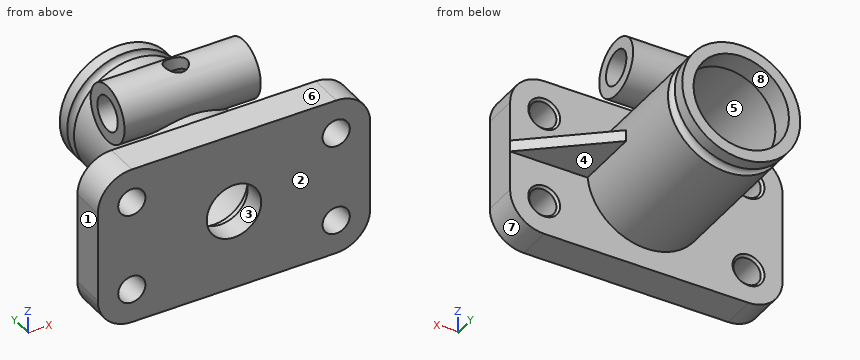
from build123d import *

# Parameters (mm, degrees)
SKETCH1_W                    = 120
SKETCH1_H                    = 70
BOSS_EXTRUDE1_DEPTH          = 15
SKETCH2_R                    = 26
BOSS_EXTRUDE2_DEPTH          = 70
SKETCH8_R                    = 2.5
BOSS_EXTRUDE3_DEPTH          = 2.5
SKETCH10_R                   = 12.5
BOSS_EXTRUDE4_DEPTH          = 60
SKETCH11_R                   = 23
CUT_EXTRUDE1_DEPTH           = 60
HOLE2_D                      = 15
SKETCH14_R                   = 5
CUT_EXTRUDE2_DEPTH           = 60
FILLET1_R                    = 15
M14_TAPPED_HOLE1_D           = 12
M14_TAPPED_HOLE1_CSINK_D     = 14.05
M14_TAPPED_HOLE1_CSINK_ANGLE = 90


with BuildPart() as part:
    # Sketch1 → Boss-Extrude1 (new body)
    with BuildSketch(Plane(origin=(0, 0, 0), x_dir=(1, 0, 0), z_dir=(0, 1, 0))):
        Rectangle(SKETCH1_W, SKETCH1_H)
    extrude(amount=BOSS_EXTRUDE1_DEPTH)

    # Sketch2 → Boss-Extrude2 (add)
    with BuildSketch(Plane(origin=(0, 15, 0), x_dir=(1, 0, 0), z_dir=(0, 1, 0))):
        with Locations(Location((0, 0, 0), (0, 0, 270))):
            Circle(SKETCH2_R)
    extrude(amount=BOSS_EXTRUDE2_DEPTH)

    # Sketch7 → Cut-Revolve2 (revolve, cut)
    with BuildSketch(Plane.XY, mode=Mode.PRIVATE) as cut_revolve2_sk:
        Polygon((0, 0), (0, 85), (21, 85), (21, 65), (23, 65), (23, 15), (15, 15), (15, 10), (12, 10), (12, 0), align=None)
    revolve(cut_revolve2_sk.sketch.rotate(Axis((0, 0, 0), (0, 1, 0)), 90), axis=Axis((0, 0, 0), (0, 1, 0)), mode=Mode.SUBTRACT)

    # Sketch8 → Cut-Revolve3 (revolve, cut)
    with BuildSketch(Plane.XY, mode=Mode.PRIVATE) as cut_revolve3_sk:
        with Locations((26, 77)):
            Circle(SKETCH8_R)
    revolve(cut_revolve3_sk.sketch.rotate(Axis((0, 0, 0), (0, 1, 0)), 90), axis=Axis((0, 0, 0), (0, 1, 0)), mode=Mode.SUBTRACT)

    # Sketch9 → Boss-Extrude3 (add, symmetric)
    with BuildSketch(Plane.XY):
        Polygon((24, 45), (60, 15), (24, 15), align=None)
    extrude(amount=BOSS_EXTRUDE3_DEPTH, both=True)

    # Sketch10 → Boss-Extrude4 (add)
    with BuildSketch(Plane(origin=(30, 0, 0), x_dir=(0, 0, -1), z_dir=(1, 0, 0))):
        with Locations((-30, 43)):
            Circle(SKETCH10_R)
    extrude(amount=-BOSS_EXTRUDE4_DEPTH)

    # Sketch11 → Cut-Extrude1 (cut)
    with BuildSketch(Plane(origin=(0, 15, 0), x_dir=(1, 0, 0), z_dir=(0, 1, 0))):
        with Locations(Location((0, 0, 0), (0, 0, 90))):
            Circle(SKETCH11_R)
    extrude(amount=CUT_EXTRUDE1_DEPTH, mode=Mode.SUBTRACT)

    # Hole2 (through all)
    with Locations(Plane(origin=(30, 0, 0), x_dir=(0, 0, -1), z_dir=(1, 0, 0))):
        with Locations((-30, 43)):
            Hole(HOLE2_D / 2)

    # Sketch14 → Cut-Extrude2 (cut)
    with BuildSketch(Plane.XY):
        with Locations(Location((0, 43, 0), (0, 0, 180))):
            Circle(SKETCH14_R)
    extrude(amount=CUT_EXTRUDE2_DEPTH, mode=Mode.SUBTRACT)

    # Fillet1
    fillet1_edges = [part.edges().sort_by_distance(p)[0] for p in [
        (-60, 7.5, -35),
        (60, 7.5, -35),
        (60, 7.5, 35),
        (-60, 7.5, 35),
    ]]
    fillet(fillet1_edges, radius=FILLET1_R)

    # M14 Tapped Hole1 (through all)
    with Locations(Plane(origin=(0, 15, 0), x_dir=(1, 0, 0), z_dir=(0, 1, 0))):
        with Locations((45, -20), (45, 20), (-45, 20), (-45, -20)):
            CounterSinkHole(M14_TAPPED_HOLE1_D / 2, M14_TAPPED_HOLE1_CSINK_D / 2, counter_sink_angle=M14_TAPPED_HOLE1_CSINK_ANGLE)


solid = part.part
Here's how the part is built. I have some questions about the finished solid (model axes, mm). Face numbers are marked on the shaded views. A direction names the side the tool comes from. Give positions to 0.01 mm unless a question says otherwise; leave off trailing zeros. Loops run counter-clockwise (first coordinate to the right, second up) from the corner with the lowest first, then second, coordinate; pieces in that order, holes last. Notation, with made-up numbers: (10, 51) -> (38, 51) arc R16 cw to (38, 72) -> close; hole circle Ø7 at (-17, -20). An arc over 180 degrees is marked (long way). One line per item, written item: value.
Q1. Suppose I cut it at B-B on z = 0. Please give me the cut outline in (x, y), then the cut area to 3 significant figures.
Answers follow:
outline: (-60, 0) -> (-12, 0) -> (-12, 10) -> (-15, 10) -> (-15, 15) -> (-23, 15) -> (-23, 75) -> (-21, 75) -> (-21, 85) -> (-26, 85) -> (-26, 79.5) arc R2.5 cw to (-26, 74.5) -> (-26, 15) -> (-60, 15) -> close; (12, 0) -> (60, 0) -> (60, 15) -> (26, 43.33) -> (26, 74.5) arc R2.5 cw to (26, 79.5) -> (26, 85) -> (21, 85) -> (21, 75) -> (23, 75) -> (23, 15) -> (15, 15) -> (15, 10) -> (12, 10) -> close
area: 2,330 mm^2
Q2. Suppose I cut it at A-A on y = 6.5. Please give me the cut outline in (x, z), then the cut area to 3 significant figures.
Answers follow:
outline: (-60, -20) arc R15 ccw to (-45, -35) -> (45, -35) arc R15 ccw to (60, -20) -> (60, 20) arc R15 ccw to (45, 35) -> (-45, 35) arc R15 ccw to (-60, 20) -> close; hole circle Ø12 at (-45, -20); hole circle Ø12 at (-45, 20); hole circle Ø24 at (0, 0); hole circle Ø12 at (45, -20); hole circle Ø12 at (45, 20)
area: 7,300 mm^2
Q3. On a 3-axis mill with a long thin cutter (end or side, diameter ignored), from which of +Z, -Z, +X, -X, +Y, -Y can I reach the whole of each face in a straight line? I mean the marked faces 4, 5, 6, 7 and 8. Say none if no direction works.
Answers follow:
face 4: -Z, +X, +Y
face 5: none
face 6: +Z, +X, -X, -Y
face 7: -Z, +X, +Y, -Y
face 8: +Y
Q4. If I drill on line 1 along Z through (x, y) = (45, 6.75); line 2 along Y through (x, z) = (7.5, 21); line 3 along X through (y, z) = (6, 0), over which ranges is the centre line in solid material (lowest first)?
Answers follow:
line 1: -35 to -26, -14 to 14, 26 to 35
line 2: 0 to 15, 75 to 85
line 3: -60 to -12, 12 to 60
Q5. We'd pull the mould along X, two halves only. Please class the marked faces 1, 2 and 3: pulls with the +X half, pulls with the -X half, needs draft (parallel to the pull), parting line crosses it, or undercut.
Answers follow:
face 1: pulls with the -X half
face 2: needs draft
face 3: undercut
Q6. Suppose I cut it at C-C on z = 30. Please give me the cut outline in (x, y), then the cut area to 3 significant figures.
Answers follow:
outline: (-56.18, 0) -> (56.18, 0) -> (56.18, 15) -> (-56.18, 15) -> close; (-30, 30.5) -> (30, 30.5) -> (30, 35.5) -> (-30, 35.5) -> close; (-30, 50.5) -> (30, 50.5) -> (30, 55.5) -> (-30, 55.5) -> close
area: 2,290 mm^2
Q7. Suppose I cut it at D-D on x = 6.5. State how many separate pieces and enclosed holes the cut face has, then the cut area to 3 significant figures.
Answers follow:
separate pieces: 2
enclosed holes: 1
area: 1,360 mm^2
Q8. I'm going to push flat-ended pins straight in: pin 1 Ø9.5 at (x, z) = (-45, 20) entering from +Y; pin 2 Ø19 at (x, z) = (45, 20) entering from +Y; pin 3 Ø3 at (y, z) = (29, -13) entering from -X; pin 4 Ø16.5 at (x, y) = (0.5, 8) entering from +Z. Where does each tip first touch, or does it pass through?
Answers follow:
pin 1: through
pin 2: y = 15
pin 3: x = -23.32
pin 4: z = 35
